Here's how the part is built. I have some questions about the finished solid (model axes, mm). Face numbers are marked on the shaded views. A direction names the side the tool comes from. Give positions to 0.01 mm unless a question says otherwise; leave off trailing zeros. Order: outer loops, then holes, each group sorted by start corner. A loop starts at its lowest first (then second) coordinate and runs counter-clockwise, first axis right, second up.
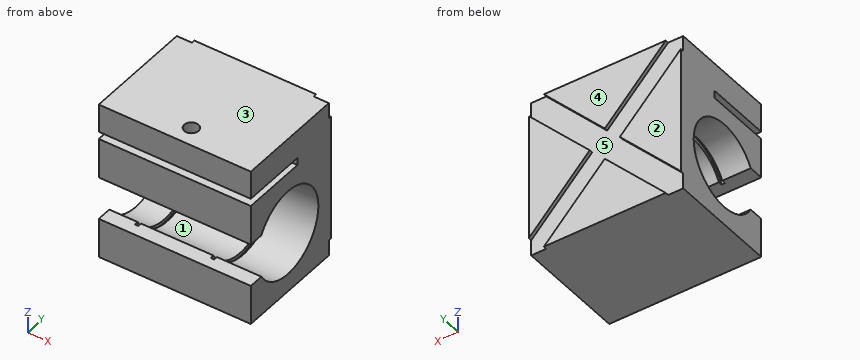
from build123d import *

# Parameters (mm, degrees)
F0_W      = 67
F0_H      = 70
F1_DEPTH  = 50
F3_DEPTH  = 1.5
F5_DEPTH  = 67
F7_R      = 20.5
F8_DEPTH  = 1.5
F9_W      = 29
F9_H      = 3.3
F10_DEPTH = 67
F12_R     = 20.5
F13_DEPTH = 1.5
F14_R     = 3.15
F15_DEPTH = 12.5


with BuildPart() as f1:
    # F0 (on Front) → F1 (new body)
    with BuildSketch(Plane.XZ):
        with Locations((-1.4453364354, 0.3557987511)):
            Rectangle(F0_W, F0_H)
    extrude(amount=F1_DEPTH)

    # F2 (on face) → F3 (cut)
    with BuildSketch(Plane(origin=(0, 0, 0), x_dir=(-1, 0, 0), z_dir=(0, 1, 0))):
        Polygon((-32.0546635646, -27.7023371982), (-32.0546635646, -34.6442012489), (-1.8768413603, -3.1151332742), (-5.199019156, 0.3557987511), align=None)
        Polygon((-1.8768413603, -3.1151332742), (-32.0546635646, -34.6442012489), (-25.4103079732, -34.6442012489), (1.4453364354, -6.5860652996), align=None)
        Polygon((-5.199019156, 0.3557987511), (-1.8768413603, -3.1151332742), (1.4453364354, 0.3557987511), (-1.8768413603, 3.8267307765), align=None)
        Polygon((1.4453364354, 0.3557987511), (-1.8768413603, -3.1151332742), (1.4453364354, -6.5860652996), (4.7675142311, -3.1151332742), align=None)
        Polygon((-1.8768413603, 3.8267307765), (1.4453364354, 0.3557987511), (4.7675142311, 3.8267307765), (1.4453364354, 7.2976628018), align=None)
        Polygon((4.7675142311, 3.8267307765), (1.4453364354, 0.3557987511), (4.7675142311, -3.1151332742), (8.0896920268, 0.3557987511), align=None)
        Polygon((-32.0546635646, 28.4139347004), (-5.199019156, 0.3557987511), (-1.8768413603, 3.8267307765), (-32.0546635646, 35.3557987511), align=None)
        Polygon((34.9453364354, 35.3557987511), (4.7675142311, 3.8267307765), (8.0896920268, 0.3557987511), (34.9453364354, 28.4139347004), align=None)
        Polygon((8.0896920268, 0.3557987511), (4.7675142311, -3.1151332742), (34.9453364354, -34.6442012489), (34.9453364354, -27.7023371982), align=None)
        Polygon((-32.0546635646, 35.3557987511), (-1.8768413603, 3.8267307765), (1.4453364354, 7.2976628018), (-25.4103079732, 35.3557987511), align=None)
        Polygon((1.4453364354, 7.2976628018), (4.7675142311, 3.8267307765), (34.9453364354, 35.3557987511), (28.300980844, 35.3557987511), align=None)
        Polygon((4.7675142311, -3.1151332742), (1.4453364354, -6.5860652996), (28.300980844, -34.6442012489), (34.9453364354, -34.6442012489), align=None)
    extrude(amount=-F3_DEPTH, mode=Mode.SUBTRACT)

    # F4 (on face) → F5 (cut, through all)
    with BuildSketch(Plane(origin=(-34.9453364354, 0, 0), x_dir=(0, -1, 0), z_dir=(-1, 0, 0))):
        with BuildLine():
            ThreePointArc((43.4544826719, 1.8557987511), (45.3525906995, -2.7266393919), (46, -7.6442012489))
            Line((46, -7.6442012489), (46.011290825, -7.6442012489))
            ThreePointArc((46.011290825, -7.6442012489), (45.3609147785, -2.7251752291), (43.4544826719, 1.8557987511))
        make_face()
        with BuildLine():
            Line((46.011290825, -7.6442012489), (46, -7.6442012489))
            ThreePointArc((46, -7.6442012489), (45.3525906995, -12.5617631058), (43.4544826719, -17.1442012489))
            ThreePointArc((43.4544826719, -17.1442012489), (45.3609147785, -12.5632272686), (46.011290825, -7.6442012489))
        make_face()
        with BuildLine():
            Line((50, 1.8557987511), (43.4544826719, 1.8557987511))
            ThreePointArc((43.4544826719, 1.8557987511), (45.3609147785, -2.7251752291), (46.011290825, -7.6442012489))
            Line((46.011290825, -7.6442012489), (50, -7.6442012489))
            Line((50, -7.6442012489), (50, 1.8557987511))
        make_face()
        with BuildLine():
            ThreePointArc((43.4544826719, -17.1442012489), (45.3525906995, -12.5617631058), (46, -7.6442012489))
            ThreePointArc((46, -7.6442012489), (45.3525906995, -2.7266393919), (43.4544826719, 1.8557987511))
            ThreePointArc((43.4544826719, 1.8557987511), (8, -7.6442012489), (43.4544826719, -17.1442012489))
        make_face()
        with BuildLine():
            ThreePointArc((46.011290825, -7.6442012489), (45.3609147785, -12.5632272686), (43.4544826719, -17.1442012489))
            Line((43.4544826719, -17.1442012489), (50, -17.1442012489))
            Line((50, -17.1442012489), (50, -7.6442012489))
            Line((50, -7.6442012489), (46.011290825, -7.6442012489))
        make_face()
    extrude(amount=-F5_DEPTH, mode=Mode.SUBTRACT)

    # F7 (on offset) → F8 (cut)
    with BuildSketch(Plane.YZ.offset(12.5)):
        with Locations((-27, -7.6442012489)):
            Circle(F7_R)
    extrude(amount=-F8_DEPTH, mode=Mode.SUBTRACT)

    # F9 (on face) → F10 (cut, through all)
    with BuildSketch(Plane(origin=(-34.9453364354, 0, 0), x_dir=(0, -1, 0), z_dir=(-1, 0, 0))):
        with Locations((35.5, 21.2057987511)):
            Rectangle(F9_W, F9_H)
    extrude(amount=-F10_DEPTH, mode=Mode.SUBTRACT)

    # F12 (on offset) → F13 (cut)
    with BuildSketch(Plane(origin=(-22.4453364354, 0, 0), x_dir=(0, -1, 0), z_dir=(-1, 0, 0))):
        with Locations((27, -7.6442012489)):
            Circle(F12_R)
    extrude(amount=-F13_DEPTH, mode=Mode.SUBTRACT)

    # F14 (on face) → F15 (cut, through all)
    with BuildSketch(Plane.XY.offset(35.3557987511)):
        with Locations((0, -41.7)):
            Circle(F14_R)
    extrude(amount=-F15_DEPTH, mode=Mode.SUBTRACT)


solid = f1.part
Q1. I need wall thicknesses on L1, parallel to Z at x = -21.45, y = -27; L2, parallel to Z at x = 13, y = -44; L3, parallel to Y at x = 0, z = 30. Which ranges of each line are inside material? Lowest first, please.
Filled sheet:
L1: z = -34.64 to -28.14, 12.86 to 19.56, 22.86 to 35.36
L2: z = -34.64 to -17.14, 1.86 to 19.56, 22.86 to 35.36
L3: y = -50 to -44.85, -38.55 to 0
Q2. If we section it at D-D on y = -41.7: Give the number of separate pieces and of enclosed holes in the cut face, plus the area to 3 significant figures.
Filled sheet:
separate pieces: 4
enclosed holes: 0
area: 2,760 mm2
Q3. If we section it at B-B on x = 0: List the corners of the cut face in (y, z) for me, plus the area to 3 significant figures.
Filled sheet:
outline: (-50, -34.64) - (0, -34.64) - (0, -8.1) - (-1.5, -8.1) - (-1.5, 8.81) - (0, 8.81) - (0, 35.36) - (-38.55, 35.36) - (-38.55, 22.86) - (-21, 22.86) - (-21, 19.56) - (-50, 19.56) - (-50, 1.86) - (-43.45, 1.86) arc R19 cw (long way) to (-43.45, -17.14) - (-50, -17.14) - close; (-50, 22.86) - (-44.85, 22.86) - (-44.85, 35.36) - (-50, 35.36) - close
area: 2,070 mm2
Q4. Thinking about a two-plate mould opening in Z: for the marked faces 1, 2 and 3, which applies, released by +Z, released by -Z, zero draft, split by the parting line, or undercut?
Filled sheet:
face 1: undercut
face 2: zero draft
face 3: released by +Z
Q5. If we section it at A-A on y = -27: List the corners of the cut face in (x, z) for me.
Filled sheet:
outline: (-34.95, -34.64) - (32.05, -34.64) - (32.05, -26.64) - (12.5, -26.64) - (12.5, -28.14) - (11, -28.14) - (11, -26.64) - (-20.95, -26.64) - (-20.95, -28.14) - (-22.45, -28.14) - (-22.45, -26.64) - (-34.95, -26.64) - close; (-34.95, 11.36) - (-22.45, 11.36) - (-22.45, 12.86) - (-20.95, 12.86) - (-20.95, 11.36) - (11, 11.36) - (11, 12.86) - (12.5, 12.86) - (12.5, 11.36) - (32.05, 11.36) - (32.05, 19.56) - (-34.95, 19.56) - close; (-34.95, 22.86) - (32.05, 22.86) - (32.05, 35.36) - (-34.95, 35.36) - close
Q6. For the marked faces 4 and 5, which set-ups out of +Z, -Z, +X, -X, +Y, -Y let a thin tool reach every point of the face, with its end or its side?
Filled sheet:
face 4: +Z, -Z, +X, -X, +Y
face 5: +Y
Q7. If we section it at C-C on z = 5: List the corners of the cut face in (x, y) for me, plus the area to 3 significant figures.
Filled sheet:
outline: (-34.95, -50) - (32.05, -50) - (32.05, -41.18) - (12.5, -41.18) - (12.5, -43.14) - (11, -43.14) - (11, -41.18) - (-20.95, -41.18) - (-20.95, -43.14) - (-22.45, -43.14) - (-22.45, -41.18) - (-34.95, -41.18) - close; (-34.95, -12.82) - (-22.45, -12.82) - (-22.45, -10.86) - (-20.95, -10.86) - (-20.95, -12.82) - (11, -12.82) - (11, -10.86) - (12.5, -10.86) - (12.5, -12.82) - (32.05, -12.82) - (32.05, 0) - (9.64, 0) - (9.64, -1.5) - (-12.53, -1.5) - (-12.53, 0) - (-34.95, 0) - close
area: 1,400 mm2
